from build123d import *

# Parameters (mm, degrees)
SKICA1_R                 = 2.6
P_IDAT_VYSUNUT_M1_DEPTH  = 2.2
SKICA2_R                 = 1.275
P_IDAT_VYSUNUT_M2_DEPTH  = 8.4
ZAOBLIT1_R               = 2
ODEBRAT_VYSUNUT_M1_DEPTH = 0.7
ZKOSEN_1_SIZE            = 0.3


with BuildPart() as part:
    # Skica1 → Přidat vysunutím1 (new body)
    with BuildSketch(Plane.XY):
        Circle(SKICA1_R)
    extrude(amount=P_IDAT_VYSUNUT_M1_DEPTH)

    # Skica2 → Přidat vysunutím2 (add)
    with BuildSketch(Plane.XY.offset(2.2)):
        Circle(SKICA2_R)
    extrude(amount=P_IDAT_VYSUNUT_M2_DEPTH)

    # Zaoblit1
    zaoblit1_edges = [part.edges().sort_by_distance(p)[0] for p in [
        (-2.6, 0, 0),
    ]]
    fillet(zaoblit1_edges, radius=ZAOBLIT1_R)

    # Skica3 → Odebrat vysunutím1 (cut)
    with BuildSketch(Plane(origin=(0, 0, 0), x_dir=(-1, 0, 0), z_dir=(0, 0, -1))):
        Polygon((-1.65, 0), (-1.65, 0.25), (-0.25, 0.25), (-0.25, 1.65), (0.25, 1.65), (0.25, 0.25), (1.65, 0.25), (1.65, -0.25), (0.25, -0.25), (0.25, -1.65), (-0.25, -1.65), (-0.25, -0.25), (-1.65, -0.25), align=None)
    extrude(amount=-ODEBRAT_VYSUNUT_M1_DEPTH, mode=Mode.SUBTRACT)

    # Zkosení1
    zkosen_1_edges = [part.edges().sort_by_distance(p)[0] for p in [
        (-1.275, 0, 10.6),
    ]]
    chamfer(zkosen_1_edges, length=ZKOSEN_1_SIZE)


solid = part.part
The model under review builds one solid part; all positions refer to its coordinate system, in mm. Round coordinates to 2 decimals unless told otherwise and drop trailing zeros. Loops run counter-clockwise (first coordinate to the right, second up) from the corner with the lowest first, then second, coordinate; pieces in that order, holes last. Notation, with made-up numbers: (-12, 16) -> (2, 16) arc R29 cw to (2, 44) -> close; hole circle Ø3 at (16.5, -38). An arc over 180 degrees is marked (long way). Answer as CSV lines item,"result".
1) For P1, Ø2, axis at x = 2, y = 1.5, coming from the -Z side; P2, Ø0.8, axis at y = -1, z = 0, coming from the -X side; P3, Ø0.6, axis at x = -1, z = 0, coming from the +Y side, all flat-tipped, find the tip position at first contact; note any pin that passes through.
Geometry results:
P1,"stops at z = 0.21"
P2,"stops at x = -1.54"
P3,"stops at y = 1.35"
2) To check wall thickness, follow line 1 along Z through (x, y) = (0.05, -0.3); line 2 along Y through (x, z) = (0.05, 4.5); line 3 along Z through (x, y) = (0.5, 0.5). State the ranges of each line that lie inside material, in increasing order. Write a range as from..to.
Geometry results:
line 1,"z = 0.7..10.6"
line 2,"y = -1.27..1.27"
line 3,"z = 0..10.6"
3) Draft analysis for pull direction X (two halves, no side actions). For faces 1 (the face through (0.59, -1.13, 6.19)), 2 (the face through (0, 0, 10.6)), 3 (the face through (0, 0, 0.7)), state which applies: pulls with the +X half, pulls with the -X half, needs draft (parallel to the pull), parting line crosses it, or undercut.
Geometry results:
face 1,"parting line crosses it"
face 2,"needs draft"
face 3,"undercut"
4) Add section A-A on z = 6.5. Write out the cut boundary in (x, y) (3 decimals), plus the area to 3 significant figures.
Geometry results:
outline,"circle Ø2.55 at (0, 0)"
area,"5.11 mm²"
